from build123d import *

# Parameters (mm, degrees)
ESQUISSE1_W             = 55
ESQUISSE1_H             = 33
BOSS_EXTRU_1_DEPTH      = 50
ENL_V_MAT_EXTRU_2_DEPTH = 45
CONG_1_R                = 5
ESQUISSE3_R             = 1.5
ENL_V_MAT_EXTRU_3_DEPTH = 10
ENL_V_MAT_EXTRU_4_DEPTH = 2


with BuildPart() as part:
    # Esquisse1 → Boss.-Extru.1 (new body)
    with BuildSketch(Plane.XY):
        with Locations((-27.5, 16.5)):
            Rectangle(ESQUISSE1_W, ESQUISSE1_H)
    extrude(amount=BOSS_EXTRU_1_DEPTH)

    # Esquisse2 → Enlèv. mat.-Extru.2 (cut)
    with BuildSketch(Plane.XY):
        with BuildLine():
            Line((-39, 29), (-16, 29))
            ThreePointArc((-16, 29), (-3, 16), (-16, 3))
            Line((-16, 3), (-39, 3))
            ThreePointArc((-39, 3), (-52, 16), (-39, 29))
        make_face()
    extrude(amount=ENL_V_MAT_EXTRU_2_DEPTH, mode=Mode.SUBTRACT)

    # Congé1
    cong_1_edges = [part.edges().sort_by_distance(p)[0] for p in [
        (0, 0, 25),
        (-55, 0, 25),
        (-55, 33, 25),
        (0, 33, 25),
    ]]
    fillet(cong_1_edges, radius=CONG_1_R)

    # Esquisse3 → Enlèv. mat.-Extru.3 (cut)
    with BuildSketch(Plane.XY.offset(50)):
        with Locations((-29, 9.3)):
            Circle(ESQUISSE3_R)
        with Locations((-9, 19.5)):
            Circle(ESQUISSE3_R)
        with Locations((-9, 9.5)):
            Circle(ESQUISSE3_R)
    extrude(amount=-ENL_V_MAT_EXTRU_3_DEPTH, mode=Mode.SUBTRACT)

    # Esquisse4 → Enlèv. mat.-Extru.4 (cut)
    with BuildSketch(Plane(origin=(0, 0, 45), x_dir=(-1, 0, 0), z_dir=(0, 0, -1))):
        Polygon((27.354551733, 6.45), (30.645448267, 6.45), (32.290896534, 9.3), (30.645448267, 12.15), (27.354551733, 12.15), (25.709103466, 9.3), align=None)
        Polygon((7.354551733, 6.65), (10.645448267, 6.65), (12.290896534, 9.5), (10.645448267, 12.35), (7.354551733, 12.35), (5.709103466, 9.5), align=None)
        Polygon((7.354551733, 16.65), (10.645448267, 16.65), (12.290896534, 19.5), (10.645448267, 22.35), (7.354551733, 22.35), (5.709103466, 19.5), align=None)
    extrude(amount=-ENL_V_MAT_EXTRU_4_DEPTH, mode=Mode.SUBTRACT)


solid = part.part
CAD build for the part. Positions are in the model's coordinates, mm. A direction names the side the tool comes from. Coordinates: 2 decimals unless noted, no trailing zeros. Order: outer loops, then holes, each group sorted by start corner. A loop starts at its lowest first (then second) coordinate and runs counter-clockwise, first axis right, second up.
Item 1: Band-saw the part on B-B on z = 10. List the corners of the cut face in (x, y).
Check sheet entries:
outline: (-55, 5) arc R5 ccw to (-50, 0) - (-5, 0) arc R5 ccw to (0, 5) - (0, 28) arc R5 ccw to (-5, 33) - (-50, 33) arc R5 ccw to (-55, 28) - close; hole (-39, 3) - (-16, 3) arc R13 ccw to (-16, 29) - (-39, 29) arc R13 ccw to start
Item 2: Band-saw the part on C-C on x = -20. List the corners of the cut face in (y, z), plus the area to 3 significant figures.
Check sheet entries:
outline: (0, 0) - (3, 0) - (3, 45) - (29, 45) - (29, 0) - (33, 0) - (33, 50) - (0, 50) - close
area: 480 mm2
Item 3: Two-plate mould, pull along Y, no slides. Class faces 3 (the face through (-27, 16, 45)), 4 (the face through (-31.48, 10.705, 45.986)), 5 (the face through (-54, 2, 25)), 6 (the face through (-28, 31, 0)): +Y half, -Y half, draft (parallel to the pull), parting line (faces both ways), or undercut.
Check sheet entries:
face 3: undercut
face 4: undercut
face 5: -Y half
face 6: draft
Item 4: 3-axis set-ups, long thin cutter, end or side, ignore diameter. For faces 1 (the face through (-10.11, 20.51, 48.52)), 2 (the face through (-6.54, 10.94, 45.99)): which of +Z, -Z, +X, -X, +Y, -Y reach the whole face in a straight line?
Check sheet entries:
face 1: +Z, -Z
face 2: -Z
Item 5: Drill centre lines: L1, parallel to Y at x = -9, z = 48.95; L2, parallel to Y at x = -30, z = 7; L3, parallel to Z at x = -7, y = 10.5. Where is each one in solid material? Low to high.
Check sheet entries:
L1: y = 0 to 8, 11 to 18, 21 to 33
L2: y = 0 to 3, 29 to 33
L3: z = 47 to 50
Item 6: Pin check, flat tips, straight feed: pin 1 Ø3 at (x, y) = (-36, 18.5) entering from -Z; pin 2 Ø1.8 at (x, y) = (-9, 9.5) entering from +Z; pin 3 Ø3.5 at (x, y) = (-9, 19.5) entering from -Z. Stop position of each tip, or through.
Check sheet entries:
pin 1: stops at z = 45
pin 2: passes through
pin 3: stops at z = 47
Item 7: Band-saw the part on D-D on x = -9. List the corners of the cut face in (y, z).
Check sheet entries:
outline: (0, 0) - (5.05, 0) - (5.05, 45) - (6.65, 45) - (6.65, 47) - (8, 47) - (8, 50) - (0, 50) - close; (11, 47) - (12.35, 47) - (12.35, 45) - (16.65, 45) - (16.65, 47) - (18, 47) - (18, 50) - (11, 50) - close; (21, 47) - (22.35, 47) - (22.35, 45) - (26.95, 45) - (26.95, 0) - (33, 0) - (33, 50) - (21, 50) - close
Item 8: Band-saw the part on A-A on x = -29. List the corners of the cut face in (y, z).
Check sheet entries:
outline: (0, 0) - (3, 0) - (3, 45) - (6.45, 45) - (6.45, 47) - (7.8, 47) - (7.8, 50) - (0, 50) - close; (10.8, 47) - (12.15, 47) - (12.15, 45) - (29, 45) - (29, 0) - (33, 0) - (33, 50) - (10.8, 50) - close
